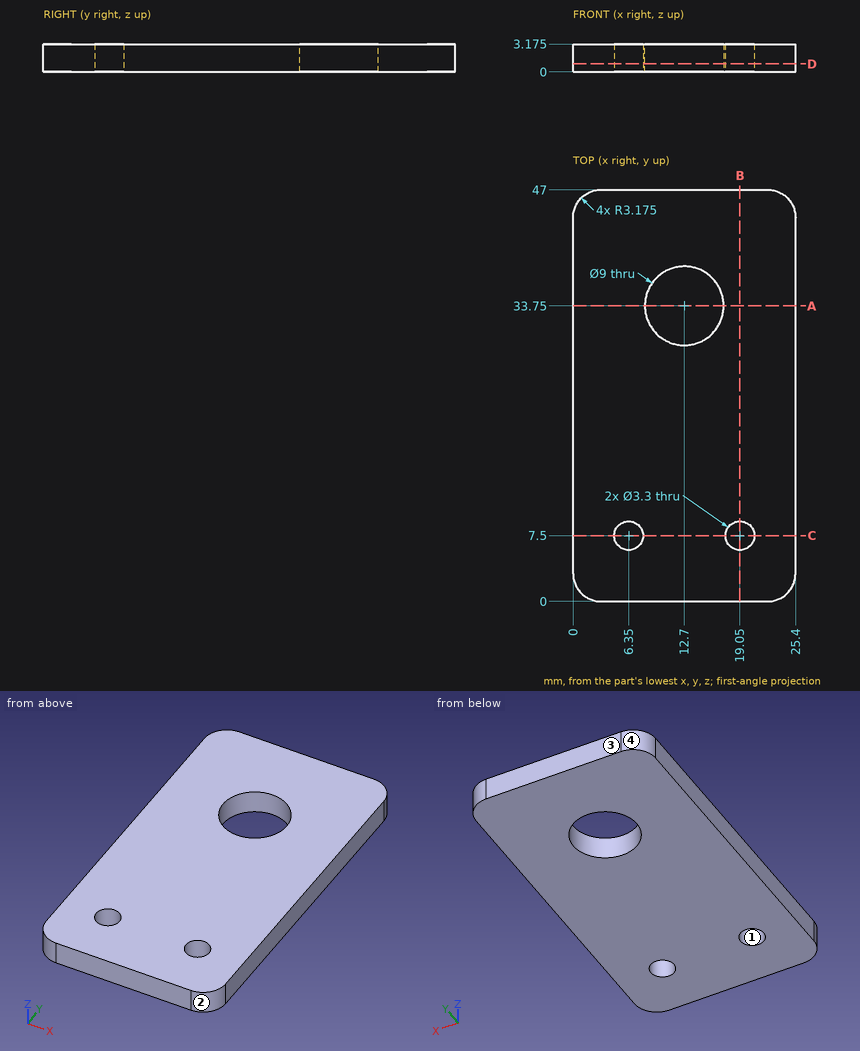
For this review, use the dimensioned drawing (mm, ordinates from the lowest corner) and the shaded views. Give positions to 0.01 mm unless a question says otherwise; leave off trailing zeros. Order: outer loops, then holes, each group sorted by start corner. A loop starts at its lowest first (then second) coordinate and runs counter-clockwise, first axis right, second up. Notation, with made-up numbers: M 14.5,-19.75 L 52.5,-19.75 A6 cw 52.5,-13.75 Z; hole C 42.5,-3 d3. An arc over 180 degrees is marked long. One line per question, with ' | ' between items. Start each with the question number.
1) Consider section C-C, the plane y = 7.5. Give the boundary of the cut face in (x, z) (3 decimals), then the cut area to 3 significant figures.
2) Consider section D-D, the plane z = 0.9. Give the boundary of the cut face in (x, y) (3 decimals).
3) Wall thickness on L1, parallel to Y at x = 12.7, z = 2.35; L2, parallel to Y at x = 6.35, z = 0.8; L3, parallel to X at y = 30.5, z = 1.7: over which ranges is each line inside the solid? List them lowest first. Write a range as from..to.
4) Consider section A-A, the plane y = 33.75. Give the boundary of the cut face in (x, z) (3 decimals), then the cut area to 3 significant figures.
5) Mouldability with a two-part tool opening along X and no side actions: class the marked faces 1, 2, 3 and 4 as pulls with the +X half, pulls with the -X half, needs draft (parallel to the pull), parting line crosses it, or undercut.
6) Consider section B-B, the plane x = 19.05. Give the boundary of the cut face in (y, z) (3 decimals).
Found:
1) outline: M 0,0 L 4.7,0 L 4.7,3.175 L 0,3.175 Z; M 8,0 L 17.4,0 L 17.4,3.175 L 8,3.175 Z; M 20.7,0 L 25.4,0 L 25.4,3.175 L 20.7,3.175 Z | area: 59.7 mm²
2) outline: M 0,3.175 A3.175 ccw 3.175,0 L 22.225,0 A3.175 ccw 25.4,3.175 L 25.4,43.825 A3.175 ccw 22.225,47 L 3.175,47 A3.175 ccw 0,43.825 Z; hole C 6.35,7.5 d3.3; hole C 12.7,33.75 d9; hole C 19.05,7.5 d3.3
3) L1: y = 0..29.25, 38.25..47 | L2: y = 0..5.85, 9.15..47 | L3: x = 0..9.59, 15.81..25.4
4) outline: M 0,0 L 8.2,0 L 8.2,3.175 L 0,3.175 Z; M 17.2,0 L 25.4,0 L 25.4,3.175 L 17.2,3.175 Z | area: 52.1 mm²
5) face 1: undercut | face 2: pulls with the +X half | face 3: needs draft | face 4: pulls with the -X half
6) outline: M 0,0 L 5.85,0 L 5.85,3.175 L 0,3.175 Z; M 9.15,0 L 47,0 L 47,3.175 L 9.15,3.175 Z
